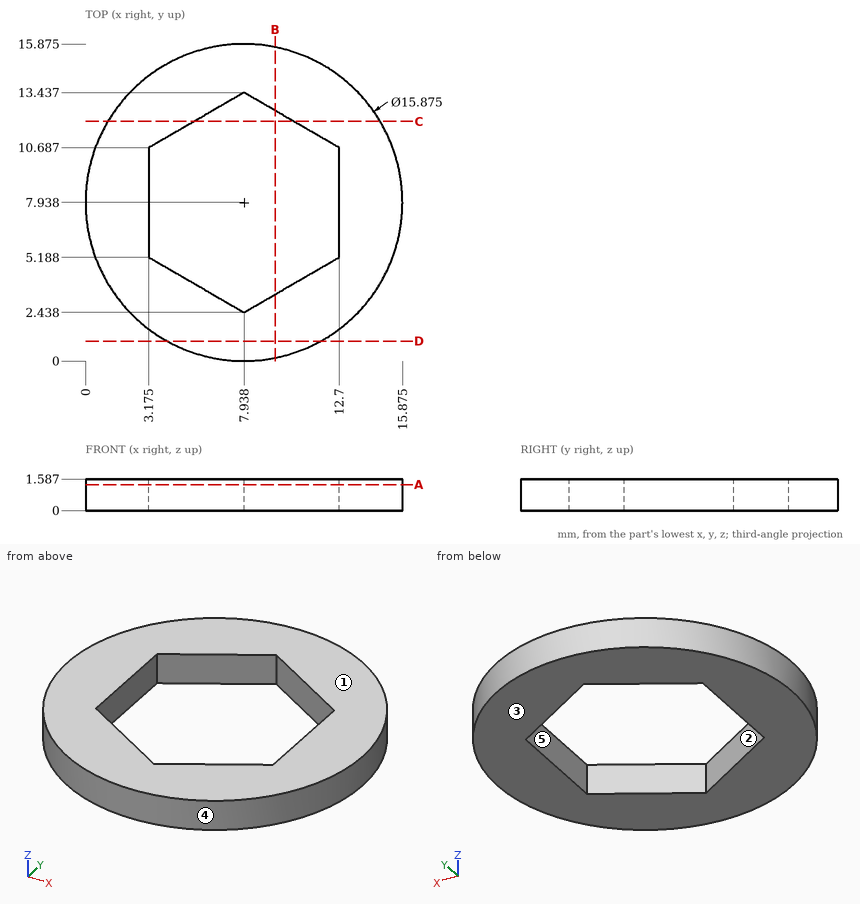
Verification items for this drawing (mm, ordinates from the low corner). A direction names the side the tool comes from. Coordinates: 2 decimals unless noted, no trailing zeros. Order: outer loops, then holes, each group sorted by start corner. A loop starts at its lowest first (then second) coordinate and runs counter-clockwise, first axis right, second up. Notation, with made-up numbers: M 22,-33.75 L 73,-33.75 A22 cw 73,4.25 Z; hole C -7.75,84.25 d3. An arc over 180 degrees is marked long. Write each question's results on one line, items separated by ' | '.
1) Section check D-D on y = 1. Record the cut outline in (x, z) (1 decimal).
Solved:
outline: M 4.1,0 L 11.8,0 L 11.8,1.6 L 4.1,1.6 Z
2) Gauge pin test, flat end, axial feed: pin 1 Ø0.8 at (y, z) = (9, 1) entering from +X. Record the tip position at first contact, or that the pin passes through.
Solved:
pin 1: stops at x = 15.85
3) Access from +Z, -Z, +X, -X, +Y, -Y to the whole of each face (thin tool, end or side, straight path). Record for the marked faces 1 and 2.
Solved:
face 1: +Z, +X, -X, +Y, -Y | face 2: +Z, -Z
4) Section check B-B on x = 9.5. Record the cut outline in (y, z) (1 decimal).
Solved:
outline: M 0.2,0 L 3.3,0 L 3.3,1.6 L 0.2,1.6 Z; M 12.5,0 L 15.7,0 L 15.7,1.6 L 12.5,1.6 Z
5) Release check for a two-part mould opening along X. For the marked faces 3, 4 and 5 record: pulls with the +X half, pulls with the -X half, needs draft (parallel to the pull), parting line crosses it, or undercut.
Solved:
face 3: needs draft | face 4: parting line crosses it | face 5: undercut
6) Section check A-A on z = 1.3. Record the cut outline in (x, y) (1 decimal), plus the area to 3 significant figures.
Solved:
outline: C 7.9,7.9 d15.9; hole M 3.2,5.2 L 7.9,2.4 L 12.7,5.2 L 12.7,10.7 L 7.9,13.4 L 3.2,10.7 Z | area: 119 mm²
7) Scan lines: line 1 along X through (y, z) = (8, 1) (1 decimal); line 2 along X through (y, z) = (9, 1.3) (1 decimal); line 3 along Y through (x, z) = (8.5, 0.6) (1 decimal). Record each from-to range of solid material in increasing order. Write a range as [from, to].
Solved:
line 1: x = [0, 3.2], [12.7, 15.9] | line 2: x = [0.1, 3.2], [12.7, 15.8] | line 3: y = [0, 2.8], [13.1, 15.9]
8) Section check C-C on y = 12. Record the cut outline in (x, z).
Solved:
outline: M 1.12,0 L 5.45,0 L 5.45,1.59 L 1.12,1.59 Z; M 10.43,0 L 14.76,0 L 14.76,1.59 L 10.43,1.59 Z
